```python
from build123d import *

# Parameters (mm, degrees)
SKETCH1_R           = 1.37499852
BOSS_EXTRUDE1_DEPTH = 3.048
SKETCH2_R           = 1.25
SKETCH2_W           = 6.7
SKETCH2_H           = 22.7542
SKETCH2_W_2         = 0.762
CUT_EXTRUDE1_DEPTH  = 4.048
SKETCH3_R           = 1.37499852
BOSS_EXTRUDE2_DEPTH = 3.048
CUT_EXTRUDE3_DEPTH  = 4.048


with BuildPart() as part:
    # Sketch1 → Boss-Extrude1 (new body)
    with BuildSketch(Plane.XY):
        with BuildLine():
            Line((0.41036367, 15.02963974), (60.10036367, 15.02963974))
            ThreePointArc((60.10036367, 15.02963974), (61.896414894, 14.285690964), (62.64036367, 12.48963974))
            Line((62.64036367, 12.48963974), (62.64036367, -38.4396361))
            ThreePointArc((62.64036367, -38.4396361), (61.896414894, -40.235687324), (60.10036367, -40.9796361))
            Line((60.10036367, -40.9796361), (0.41036367, -40.9796361))
            ThreePointArc((0.41036367, -40.9796361), (-1.385687554, -40.235687324), (-2.12963633, -38.4396361))
            Line((-2.12963633, -38.4396361), (-2.12963633, 12.48963974))
            ThreePointArc((-2.12963633, 12.48963974), (-1.385687554, 14.285690964), (0.41036367, 15.02963974))
        make_face()
        with Locations((1.37500106, 11.52500108)):
            Circle(SKETCH1_R, mode=Mode.SUBTRACT)
        with Locations((59.3750019, 11.52500108)):
            Circle(SKETCH1_R, mode=Mode.SUBTRACT)
        with Locations((59.3750019, -37.47499998)):
            Circle(SKETCH1_R, mode=Mode.SUBTRACT)
        with Locations((1.37500106, -37.47499998)):
            Circle(SKETCH1_R, mode=Mode.SUBTRACT)
    extrude(amount=-BOSS_EXTRUDE1_DEPTH)

    # Sketch2 → Cut-Extrude1 (cut, through all)
    with BuildSketch(Plane.XY):
        with Locations((29.315152151, -2.00169818)):
            Circle(SKETCH2_R)
        with Locations((41.838752151, -2.00169818)):
            Circle(SKETCH2_R)
        with Locations((41.838752151, -23.57459818)):
            Circle(SKETCH2_R)
        with Locations((29.315152151, -23.57459818)):
            Circle(SKETCH2_R)
        with Locations((23.210252151, -12.97499818)):
            Rectangle(SKETCH2_W, SKETCH2_H)
        with Locations((14.399252151, -12.97499818)):
            Rectangle(SKETCH2_W_2, SKETCH2_H)
    extrude(amount=-CUT_EXTRUDE1_DEPTH, mode=Mode.SUBTRACT)

    # Sketch3 → Boss-Extrude2 (add, through all)
    with BuildSketch(Plane.XY):
        with BuildLine():
            Line((-80.129638806, 12.489638674), (-80.129638806, -38.439637166))
            ThreePointArc((-80.129638806, -38.439637166), (-79.38569003, -40.23568839), (-77.589638806, -40.979637166))
            Line((-77.589638806, -40.979637166), (2.339634914, -40.979637166))
            ThreePointArc((2.339634914, -40.979637166), (4.135686138, -40.23568839), (4.879634914, -38.439637166))
            Line((4.879634914, -38.439637166), (4.879634914, 12.489638674))
            ThreePointArc((4.879634914, 12.489638674), (4.135686138, 14.285689898), (2.339634914, 15.029638674))
            Line((2.339634914, 15.029638674), (-77.589638806, 15.029638674))
            ThreePointArc((-77.589638806, 15.029638674), (-79.38569003, 14.285689898), (-80.129638806, 12.489638674))
        make_face()
        with Locations((1.37500106, -37.47499998)):
            Circle(SKETCH3_R, mode=Mode.SUBTRACT)
        with Locations((-56.62499978, -37.47499998)):
            Circle(SKETCH3_R, mode=Mode.SUBTRACT)
        with Locations((-56.62499978, 11.52500108)):
            Circle(SKETCH3_R, mode=Mode.SUBTRACT)
        with Locations((1.37500106, 11.52500108)):
            Circle(SKETCH3_R, mode=Mode.SUBTRACT)
    extrude(amount=-BOSS_EXTRUDE2_DEPTH)

    # Sketch5 → Cut-Extrude3 (cut, through all)
    with BuildSketch(Plane(origin=(0, 0, -3.048), x_dir=(-1, 0, 0), z_dir=(0, 0, -1))):
        with BuildLine():
            Line((-1.37500106, 15.02963974), (-32.538255274, 10.806103009))
            ThreePointArc((-32.538255274, 10.806103009), (-53.314152149, -12.975840892), (-32.537536563, -36.757156908))
            Line((-32.537536563, -36.757156908), (-1.37500106, -40.979637166))
            Line((-1.37500106, -40.979637166), (-97.655992842, -40.979637166))
            Line((-97.655992842, -40.979637166), (-97.655992842, 15.02963974))
            Line((-97.655992842, 15.02963974), (-1.37500106, 15.02963974))
        make_face()
    extrude(amount=-CUT_EXTRUDE3_DEPTH, mode=Mode.SUBTRACT)


solid = part.part
```
CAD build for the part. Positions are in the model's coordinates, mm. A direction names the side the tool comes from. Coordinates: 2 decimals unless noted, no trailing zeros. Write each loop counter-clockwise with the first axis right and the second up, starting at its lowest first coordinate (ties: lowest second). Pieces come first, ordered by that corner, then holes.
(1) Cut at D-D, the plane y = -28. List the corners of the cut face in (x, z).
(2) Flat gauge pins, fed straight in: pin 1 (0.8 mm diameter, centred on x = 14.5, z = -2, fed in from -Y); pin 2 (0.9 mm diameter, centred on y = -18, z = -1, fed in from +X); pin 3 (0.9 mm diameter, centred on y = -15, z = -1.5, fed in from +X). Where does each tip first touch, or does it go through?
(3) 3-axis set-ups, long thin cutter, end or side, ignore diameter. For faces 4 (the face through (-79.366, 14.305, -1.503)), 5 (the face through (23, -1.598, -2)): which of +Z, -Z, +X, -X, +Y, -Y reach the whole face in a straight line?
(4) Cut at C-C, the plane x = 37. List the corners of the cut face in (y, z), and give its area (3 significant figures).
(5) Cut at A-A, the plane y = -13.5. List the corners of the cut face in (x, z), and give its area (3 significant figures).
(6) Cut at B-B, the plane z = -2.4. Count the separate pieces of the cut face and the enclosed holes in it, and give its area (3 significant figures).
(7) Two-plate mould, pull along X, no slides. Class faces 1 (the face through (23, -24.352, -2)), 2 (the face through (-39, -40.98, -2)), 3 (the face through (16.738, 12.947, -1.545)): +X half, -X half, draft (parallel to the pull), parting line (faces both ways), or undercut.
(8) Drill centre lines: probe 1 along X at (y, z) = (-3.5, -2.1); probe 2 along X at (y, z) = (-23.5, -2.8); probe 3 along X at (y, z) = (-24, -2.75). Where is each one in solid material? Low to high.
Geometry says:
1. outline: (-80.13, -3.05) - (48.03, -3.05) - (48.03, 0) - (-80.13, 0) - close
2. pin 1: stops at y = -39.26
2. pin 2: stops at x = 52.87
2. pin 3: stops at x = 53.26
3. face 4: +Z, -Z, -X, +Y
3. face 5: +Z, -Z
4. outline: (-35.71, -3.05) - (9.76, -3.05) - (9.76, 0) - (-35.71, 0) - close
4. area: 139 mm2
5. outline: (-80.13, -3.05) - (14.02, -3.05) - (14.02, 0) - (-80.13, 0) - close; (14.78, -3.05) - (19.86, -3.05) - (19.86, 0) - (14.78, 0) - close; (26.56, -3.05) - (53.31, -3.05) - (53.31, 0) - (26.56, 0) - close
5. area: 384 mm2
6. separate pieces: 1
6. enclosed holes: 10
6. area: 6,710 mm2
7. face 1: undercut
7. face 2: draft
7. face 3: +X half
8. probe 1: x = -80.13 to 14.02, 14.78 to 19.86, 26.56 to 51.36
8. probe 2: x = -80.13 to 14.02, 14.78 to 19.86, 26.56 to 28.07, 30.56 to 40.59, 43.09 to 50.88
8. probe 3: x = -80.13 to 14.02, 14.78 to 19.86, 26.56 to 28.14, 30.49 to 40.66, 43.01 to 50.63
